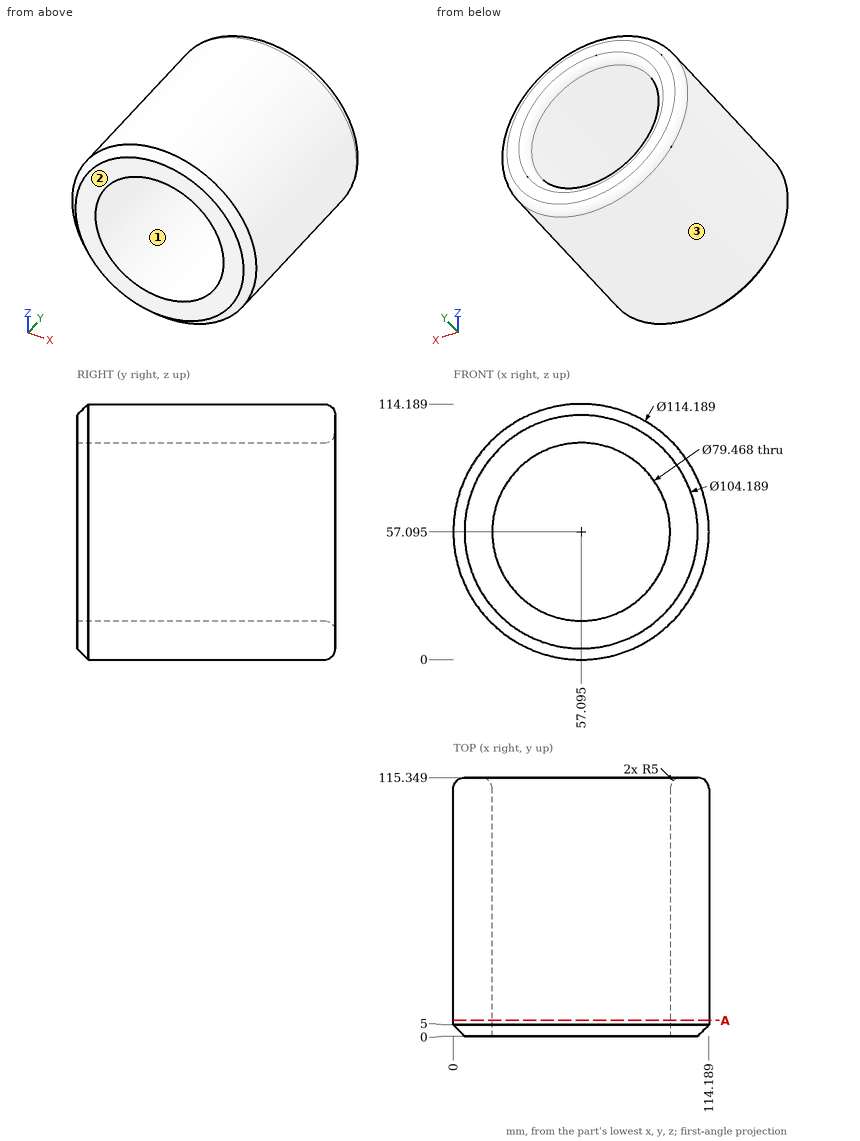
Check sheet for the drawn part. Datum: minimum x, y, z corner. Units: mm. Round coordinates to 2 decimals unless told otherwise and drop trailing zeros. Order: outer loops, then holes, each group sorted by start corner. A loop starts at its lowest first (then second) coordinate and runs counter-clockwise, first axis right, second up. Notation, with made-up numbers: M 60,23.5 L 65,23.5 A29 ccw 65,57.5 Z; hole C 84.25,66.5 d5. An arc over 180 degrees is marked long. Write each question's results on one line, items separated by ' | '. Start each with the question number.
1. Cross-section at A-A on y = 7. Record the boundary of the cut face in (x, z) (1 decimal).
2. Draft check along X on the marked faces 1, 2 and 3. Enter one of: pulls with the +X half, pulls with the -X half, needs draft (parallel to the pull), parting line crosses it, or undercut.
3. Material ranges on L1, parallel to X at y = 75, z = 56.5 (1 decimal); L2, parallel to Z at x = 42, y = 100.5; L3, parallel to X at y = 74, z = 52, recorded low to high. Write a range as from..to.
4. Go/stop test with flat-tipped pins: P1, Ø4, axis at x = 95.5, y = 90, coming from the -Z side; P2, Ø1, axis at x = 74, z = 20.5, coming from the -Y side; P3, Ø10, axis at y = 51, z = 88.5, coming from the +X side; P4, Ø3, axis at x = 16.5, y = 91.5, coming from the -Z side (1 decimal). Record where each tip stops, or that it passes through.
Resolved:
1) outline: C 57.1,57.1 d114.2; hole C 57.1,57.1 d79.5
2) face 1: undercut | face 2: needs draft | face 3: parting line crosses it
3) L1: 0..17.4, 96.8..114.2 | L2: 2.03..20.34, 93.85..112.16 | L3: 0.23..17.69, 96.5..113.96
4) P1: z = 13.11 | P2: y = 0 | P3: x = 107.72 | P4: z = 15.5
